The listing builds one solid part. Answer for the finished solid, in the listing's coordinates (mm). Face numbers are marked on the shaded views. A direction names the side the tool comes from. Round coordinates to 2 decimals unless told otherwise and drop trailing zeros. Order: outer loops, then holes, each group sorted by start corner. A loop starts at its lowest first (then second) coordinate and runs counter-clockwise, first axis right, second up. Notation, with made-up numbers: (35.25, 19.25) -> (81.25, 19.25) arc R6 ccw to (81.25, 26.25) -> close; hole circle Ø4 at (-15.75, 24). An arc over 180 degrees is marked (long way). Return JSON: item names as keys, results as strings. Group by question number.
(1) Consider line 1 (X direction, y = 3.25, z = -37.5); line 2 (Z direction, x = 4.5, y = 61.5); line 3 (Y direction, x = -40, z = 8). Determine where each line is inside the solid, lowest interval first. Write a range as [from, to].
(2) Each of these flat-tipped pins is pushed along its axis until it touches: pin 1 (8 mm diameter, centred on x = -15, z = 22.5, fed in from +Y); pin 2 (1.5 mm diameter, centred on x = -14.5, y = 6, fed in from -Z); pin 3 (1.2 mm diameter, centred on y = 39, z = 78, fed in from +X). Where does it stop, or does it pass through?
(3) The part is cut by section A-A (y = 49). Determine the outline of the cut face in (x, z), plus the area to 3 significant figures.
(4) The part is cut by section B-B (z = 0). Determine the outline of the cut face in (x, y), plus the area to 3 significant figures.
(5) The part is cut by section C-C (x = 23). Determine the outline of the cut face in (y, z).
(6) Which of the six approach directions +Z, -Z, +X, -X, +Y, -Y give full straight-line access (tool end or side, diameter ignored) to the marked faces 3, 4 and 5?
(7) The part is cut by section D-D (x = -36). Determine the outline of the cut face in (y, z), plus the area to 3 significant figures.
(8) Determine the mould class of the marked faces 1 and 2 for opening direction X: +X half, -X half, draft (parallel to the pull), parting line (faces both ways), or undercut.
from build123d import *

# Parameters (mm, degrees)
SKETCH_1_W          = 87
SKETCH_1_H          = 90
SKETCH_1_R          = 3
SKETCH_1_H_2        = 35
EXTRUDE_1_DEPTH     = 4
SKETCH_3_W          = 87
SKETCH_3_H          = 60
SKETCH_3_R          = 17.5
EXTRUDE_2_DEPTH     = 3
SKETCH_4_R          = 2
CUT_EXTRUDE_1_DEPTH = 92.149602303
SKETCH_5_W          = 50
SKETCH_5_H          = 60
SKETCH_5_R          = 8.1
EXTRUDE_3_DEPTH     = 4


with BuildPart() as part:
    # 草图1 → 凸台-拉伸1 (new body)
    # profile 1 of 2: a face of its own
    with BuildSketch(Plane(origin=(0, 0, 0), x_dir=(1, 0, 0), z_dir=(0, 1, 0))):
        Rectangle(SKETCH_1_W, SKETCH_1_H)
        with Locations(Location((36, 37.5, 0), (0, 0, 270))):
            Circle(SKETCH_1_R, mode=Mode.SUBTRACT)
        with Locations(Location((-36, 37.5, 0), (0, 0, 270))):
            Circle(SKETCH_1_R, mode=Mode.SUBTRACT)
        with Locations(Location((36, -37.5, 0), (0, 0, 270))):
            Circle(SKETCH_1_R, mode=Mode.SUBTRACT)
        with Locations(Location((-36, -37.5, 0), (0, 0, 270))):
            Circle(SKETCH_1_R, mode=Mode.SUBTRACT)
    # profile 2 of 2: a face of its own
    with BuildSketch(Plane(origin=(0, 0, 0), x_dir=(1, 0, 0), z_dir=(0, 1, 0))):
        with Locations((0, -62.5)):
            Rectangle(SKETCH_1_W, SKETCH_1_H_2)
    extrude(amount=EXTRUDE_1_DEPTH)

    # 草图3 → 凸台-拉伸2 (add)
    with BuildSketch(Plane(origin=(0, 4, 0), x_dir=(1, 0, 0), z_dir=(0, 1, 0))):
        Rectangle(SKETCH_3_W, SKETCH_3_H)
        with Locations(Location((-23, 0, 0), (0, 0, 270))):
            Circle(SKETCH_3_R, mode=Mode.SUBTRACT)
        with Locations(Location((23, 0, 0), (0, 0, 270))):
            Circle(SKETCH_3_R, mode=Mode.SUBTRACT)
    extrude(amount=EXTRUDE_2_DEPTH)

    # 草图4 → 切除-拉伸1 (cut, through all)
    with BuildSketch(Plane(origin=(0, 4, 0), x_dir=(1, 0, 0), z_dir=(0, 1, 0))):
        with Locations(Location((23, 0, 0), (0, 0, 270))):
            Circle(SKETCH_4_R)
        with Locations(Location((-23, 0, 0), (0, 0, 270))):
            Circle(SKETCH_4_R)
    extrude(amount=-CUT_EXTRUDE_1_DEPTH, mode=Mode.SUBTRACT)

    # 草图5 → 凸台-拉伸3 (add)
    with BuildSketch(Plane.XY.offset(80)):
        with Locations((0, 34)):
            Rectangle(SKETCH_5_W, SKETCH_5_H)
        with Locations((0, 49)):
            Circle(SKETCH_5_R, mode=Mode.SUBTRACT)
    extrude(amount=-EXTRUDE_3_DEPTH)


solid = part.part
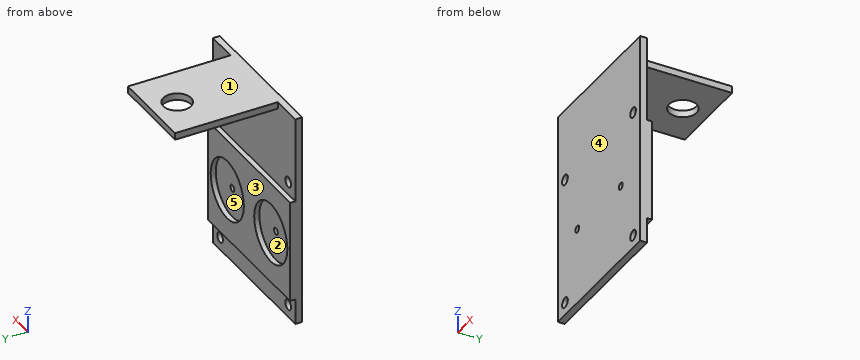
Answer below:
{
 "1": {"line 1": "x = [-43.5, -39], [-33, 33], [39, 43.5]", "line 2": "z = [76, 80]", "line 3": "y = [0, 7]"},
 "2": {"pin 1": "stops at y = 7", "pin 2": "stops at z = -30", "pin 3": "stops at x = 25"},
 "3": {"outline": "(-25, 76) -> (-8.1, 76) -> (-8.1, 80) -> (-25, 80) -> close; (8.1, 76) -> (25, 76) -> (25, 80) -> (8.1, 80) -> close", "area": "135 mm²"},
 "4": {"outline": "(-43.5, 0) -> (-25, 0) -> (-25, 4) -> (-40.5, 4) -> (-40.5, 7) -> (-43.5, 7) -> close; (-21, 0) -> (21, 0) -> (21, 4) -> (5.5, 4) -> (5.5, 7) -> (-5.5, 7) -> (-5.5, 4) -> (-21, 4) -> close; (25, 0) -> (43.5, 0) -> (43.5, 7) -> (40.5, 7) -> (40.5, 4) -> (25, 4) -> close", "area": "367 mm²"},
 "5": {"outline": "(0, -45) -> (4, -45) -> (4, -30) -> (7, -30) -> (7, -17.5) -> (4, -17.5) -> (4, -2) -> (0, -2) -> close; (0, 2) -> (4, 2) -> (4, 17.5) -> (7, 17.5) -> (7, 30) -> (4, 30) -> (4, 76) -> (64, 76) -> (64, 80) -> (0, 80) -> close"},
 "6": {"face 3": "-Z, +X, -X, +Y", "face 4": "+Z, -Z, +X, -X, -Y", "face 5": "+Y"},
 "7": {"outline": "(0, -45) -> (4, -45) -> (4, -40.5) -> (0, -40.5) -> close; (0, -34.5) -> (4, -34.5) -> (4, -30) -> (7, -30) -> (7, -11.72) -> (4, -11.72) -> (4, 11.72) -> (7, 11.72) -> (7, 30) -> (4, 30) -> (4, 34.5) -> (0, 34.5) -> close; (0, 40.5) -> (4, 40.5) -> (4, 80) -> (0, 80) -> close", "area": "562 mm²"},
 "8": {"face 1": "draft", "face 2": "undercut"}
}
